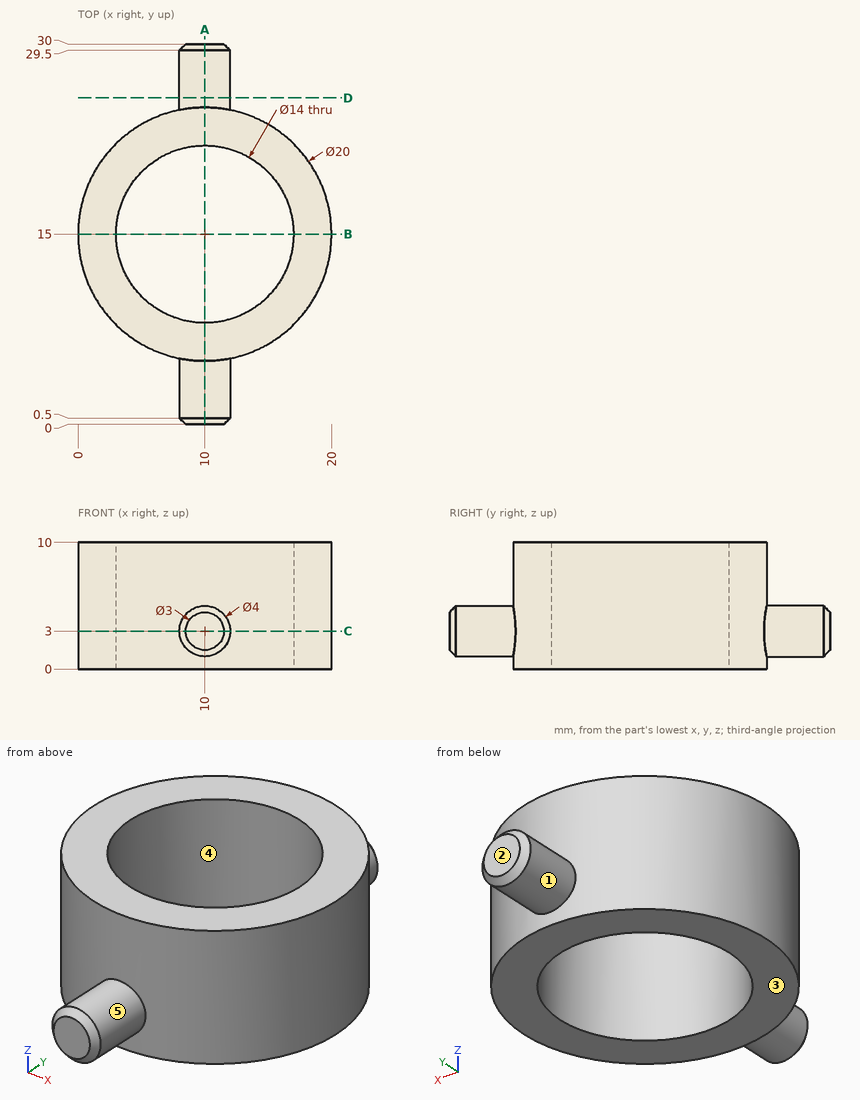
Geometry: see drawing. Coordinates: mm, zero at the bounding-box minimum. A direction names the side the tool comes from. Coordinates: 2 decimals unless noted, no trailing zeros. Loops run counter-clockwise (first coordinate to the right, second up) from the corner with the lowest first, then second, coordinate; pieces in that order, holes last. Notation, with made-up numbers: M -16.75,55 L 19.25,55 A6 cw 19.25,62 Z; hole C 17.25,-2.5 d9. An arc over 180 degrees is marked long. Answer in a Markdown table with one row per item.
Q1. Section A-A on x = 10. Return the cut outline in (y, z), plus the area to 3 significant figures.
Answers below:
| item | result |
|---|---|
| outline | M 0,1.5 L 0.5,1 L 5,1 L 5,0 L 8,0 L 8,10 L 5,10 L 5,5 L 0.5,5 L 0,4.5 Z; M 22,0 L 25,0 L 25,1 L 29.5,1 L 30,1.5 L 30,4.5 L 29.5,5 L 25,5 L 25,10 L 22,10 Z |
| area | 99.5 mm^2 |
Q2. Set-up query: the marked faces 1 and 2. Return all of +Z, -Z, +X, -X, +Y, -Y with unobstructed straight access to the full face (end or side cutting, diameter ignored); none if empty.
Answers below:
| item | result |
|---|---|
| face 1 | +Y |
| face 2 | +Z, -Z, +X, -X, +Y |
Q3. Section C-C on z = 3. Return the cut outline in (x, y).
Answers below:
| item | result |
|---|---|
| outline | M 8,0.5 L 8.5,0 L 11.5,0 L 12,0.5 L 12,5.2 A10 ccw 12,24.8 L 12,29.5 L 11.5,30 L 8.5,30 L 8,29.5 L 8,24.8 A10 ccw 8,5.2 Z; hole C 10,15 d14 |
Q4. Section B-B on y = 15. Return the cut outline in (x, z), plus the area to 3 significant figures.
Answers below:
| item | result |
|---|---|
| outline | M 0,0 L 3,0 L 3,10 L 0,10 Z; M 17,0 L 20,0 L 20,10 L 17,10 Z |
| area | 60.0 mm^2 |
Q5. Section D-D on y = 25.75. Return the cut outline in (x, z), plus the area to 3 significant figures.
Answers below:
| item | result |
|---|---|
| outline | C 10,3 d4 |
| area | 12.6 mm^2 |
Q6. Ray query, probe 1 along Y at (x, z) = (10, 2.25); probe 2 along Y at (x, z) = (10.25, 8.25); probe 3 along X at (y, z) = (17, 6.5). Return the intervals inside material, ascending. Write a range as from..to.
Answers below:
| item | result |
|---|---|
| probe 1 | y = 0..8, 22..30 |
| probe 2 | y = 5..8, 22..25 |
| probe 3 | x = 0.2..3.29, 16.71..19.8 |
Q7. Draft query along X for the marked faces 3, 4 and 5. Return one class per face: pulls with the +X half, pulls with the -X half, needs draft (parallel to the pull), parting line crosses it, or undercut.
Answers below:
| item | result |
|---|---|
| face 3 | needs draft |
| face 4 | undercut |
| face 5 | parting line crosses it |
Q8. First-contact query: pin 1 (1 mm diameter, centred on y = 7, z = 6, fed in from -X); pin 2 (2 mm diameter, centred on y = 20, z = 6.5, fed in from +X); pin 3 (2 mm diameter, centred on x = 15, z = 1, fed in from +Y). Flat tips, straight axial feed; report the tip coordinate or a pass-through.
Answers below:
| item | result |
|---|---|
| pin 1 | stops at x = 3.39 |
| pin 2 | stops at x = 19.17 |
| pin 3 | stops at y = 24.17 |
